Answer from the drawing. Dimensions are ordinates in mm from the lowest x, y and z of the part. A direction names the side the tool comes from. Round coordinates to 2 decimals unless told otherwise and drop trailing zeros. Loops run counter-clockwise (first coordinate to the right, second up) from the corner with the lowest first, then second, coordinate; pieces in that order, holes last.
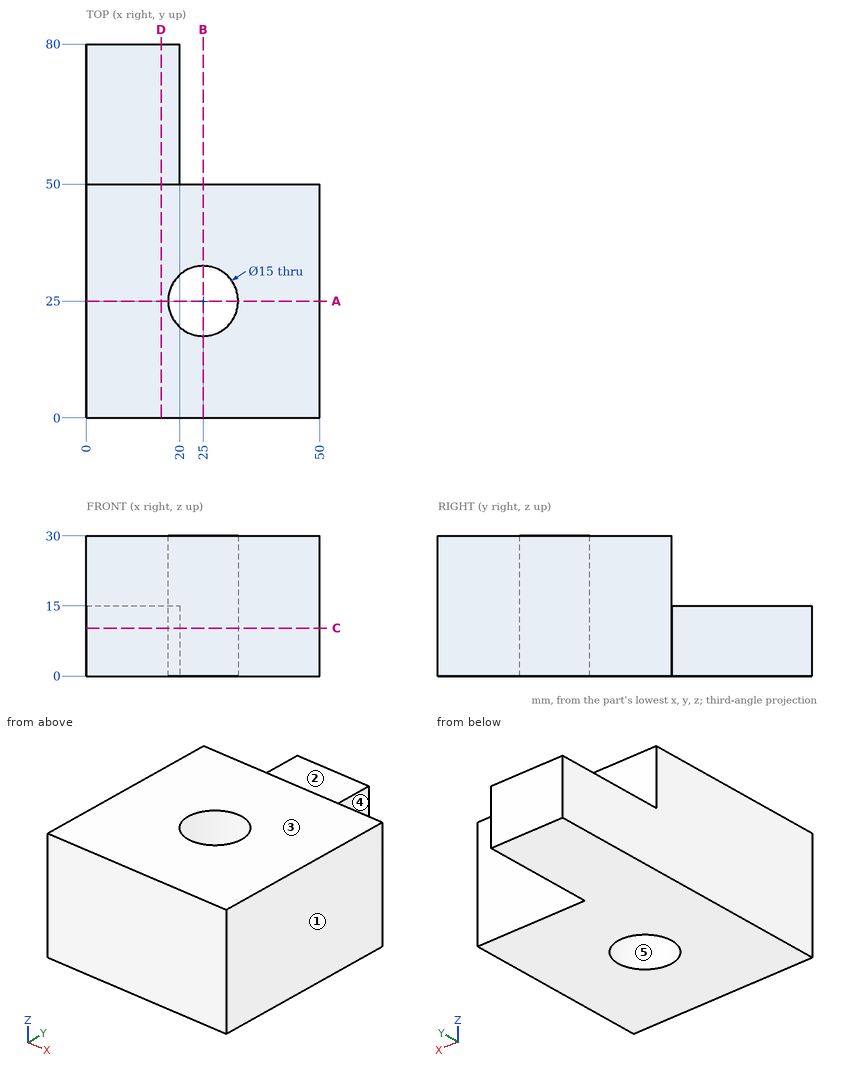
1. Consider probe 1 along Y at (x, z) = (25, 8); probe 2 along Y at (x, z) = (34.5, 20); probe 3 along X at (y, z) = (65, 12). Determine where each line is inside the solid, lowest interval first.
Answer key:
probe 1: y = 0 to 17.5, 32.5 to 50
probe 2: y = 0 to 50
probe 3: x = 0 to 20
2. Find section C-C (z = 10.25). Write down the section's boundary in (x, y), then the cut area to 3 significant figures.
Answer key:
outline: (0, 0) - (50, 0) - (50, 50) - (20, 50) - (20, 80) - (0, 80) - close; hole circle Ø15 at (25, 25)
area: 2,920 mm2
3. Find section A-A (y = 25). Write down the section's boundary in (x, z), then the cut area to 3 significant figures.
Answer key:
outline: (0, 0) - (17.5, 0) - (17.5, 30) - (0, 30) - close; (32.5, 0) - (50, 0) - (50, 30) - (32.5, 30) - close
area: 1,050 mm2
4. Find section D-D (x = 16). Write down the section's boundary in (y, z), then the cut area to 3 significant figures.
Answer key:
outline: (0, 0) - (80, 0) - (80, 15) - (50, 15) - (50, 30) - (0, 30) - close
area: 1,950 mm2
5. Determine the mould class of the marked faces 3, 4 and 5 for opening direction X: +X half, -X half, draft (parallel to the pull), parting line (faces both ways), or undercut.
Answer key:
face 3: draft
face 4: +X half
face 5: undercut
6. Which of the six approach directions +Z, -Z, +X, -X, +Y, -Y give full straight-line access (tool end or side, diameter ignored) to the marked faces 1 and 2?
Answer key:
face 1: +Z, -Z, +X, +Y, -Y
face 2: +Z, +X, -X, +Y
7. Given pin 1 (7.5 mm diameter, centred on y = 60.5, z = 9.5, fed in from +X); pin 2 (16 mm diameter, centred on x = 10.5, y = 61, fed in from +Z); pin 3 (12 mm diameter, centred on x = 40, z = 7, fed in from +Y), each flat-ended and moving along its own axis, determine where each tip first touches the part or whether it passes through.
Answer key:
pin 1: stops at x = 20
pin 2: stops at z = 15
pin 3: stops at y = 50
